```python
from build123d import *

# Parameters (mm, degrees)
SKETCH1_R           = 10.8
BOSS_EXTRUDE1_DEPTH = 5.08
SKETCH2_R           = 9.45
BOSS_EXTRUDE2_DEPTH = 2.54
CUT_EXTRUDE1_DEPTH  = 18.068813667


with BuildPart() as part:
    # Sketch1 → Boss-Extrude1 (new body)
    with BuildSketch(Plane.XY):
        Circle(SKETCH1_R)
    extrude(amount=BOSS_EXTRUDE1_DEPTH)

    # Sketch2 → Boss-Extrude2 (add)
    with BuildSketch(Plane.XY.offset(5.08)):
        Circle(SKETCH2_R)
    extrude(amount=BOSS_EXTRUDE2_DEPTH)

    # Sketch3 → Cut-Extrude1 (cut, through all)
    with BuildSketch(Plane.XY.offset(7.62)):
        with BuildLine():
            Line((-2, 0), (-2, 2.236067977))
            ThreePointArc((-2, 2.236067977), (3, 0), (-2, -2.236067977))
            Line((-2, -2.236067977), (-2, 0))
        make_face()
    extrude(amount=-CUT_EXTRUDE1_DEPTH, mode=Mode.SUBTRACT)


solid = part.part
```
The listing builds one solid part. Answer for the finished solid, in the listing's coordinates (mm). A direction names the side the tool comes from. Coordinates: 2 decimals unless noted, no trailing zeros. Write each loop counter-clockwise with the first axis right and the second up, starting at its lowest first coordinate (ties: lowest second). Pieces come first, ordered by that corner, then holes.
Q1. Given P1, Ø3, axis at y = 5, z = 6, coming from the -X side, flat-ended and moving along its own axis, determine where the tip first touches the part or whether it passes through.
Returned:
P1: stops at x = -10.1
Q2. Which of the six approach directions +Z, -Z, +X, -X, +Y, -Y give full straight-line access (tool end or side, diameter ignored) to faces 1 (the cylindrical face through (9.014, 2.839, 6.332)), 2 (the flat face through (-2.2, 0.1, 7.62))?
Returned:
face 1: +Z
face 2: +Z, +X, -X, +Y, -Y
Q3. Section D-D, the plane x = -8 is taken. Write down the section's boundary in (y, z), then the cut area to 3 significant figures.
Returned:
outline: (-7.26, 0) - (7.26, 0) - (7.26, 5.08) - (5.03, 5.08) - (5.03, 7.62) - (-5.03, 7.62) - (-5.03, 5.08) - (-7.26, 5.08) - close
area: 99.3 mm2
Q4. Section A-A, the plane y = 0 is taken. Write down the section's boundary in (x, z).
Returned:
outline: (-10.8, 0) - (-2, 0) - (-2, 7.62) - (-9.45, 7.62) - (-9.45, 5.08) - (-10.8, 5.08) - close; (3, 0) - (10.8, 0) - (10.8, 5.08) - (9.45, 5.08) - (9.45, 7.62) - (3, 7.62) - close
Q5. Section C-C, the plane z = 6.25 is taken. Write down the section's boundary in (x, y), then the cut area to 3 significant figures.
Returned:
outline: circle Ø18.9 at (0, 0); hole (-2, -2.24) arc R3 ccw (long way) to (-2, 2.24) - close
area: 255 mm2
Q6. The mould has two halves that part along X. Classify faces 3 (the flat face through (-3, 0, 0)), 4 (the cylindrical face through (-2.341, -10.543, 2.504)), 5 (the flat face through (-2, 0, 4)): released by +X, released by -X, zero draft, split by the parting line, or undercut.
Returned:
face 3: zero draft
face 4: split by the parting line
face 5: undercut
Q7. Section B-B, the plane x = 0 is taken. Write down the section's boundary in (y, z).
Returned:
outline: (-10.8, 0) - (-3, 0) - (-3, 7.62) - (-9.45, 7.62) - (-9.45, 5.08) - (-10.8, 5.08) - close; (3, 0) - (10.8, 0) - (10.8, 5.08) - (9.45, 5.08) - (9.45, 7.62) - (3, 7.62) - close
Q8. Find the intervals of material crossed by line 1 along Y through (x, z) = (0, 2.5); line 2 along X through (y, z) = (2.25, 1); line 3 along X through (y, z) = (-0.5, 6.75), in increasing order.
Returned:
line 1: y = -10.8 to -3, 3 to 10.8
line 2: x = -10.56 to -1.98, 1.98 to 10.56
line 3: x = -9.44 to -2, 2.96 to 9.44
